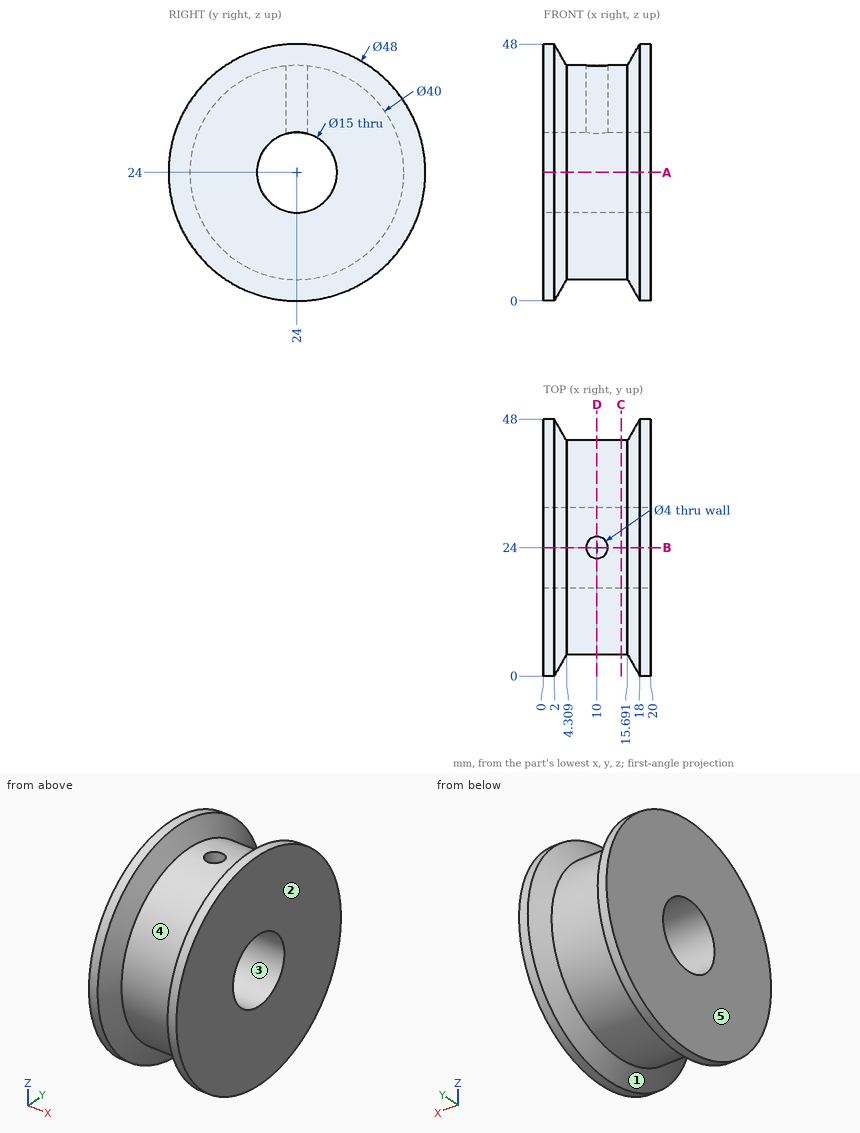
Answer from the drawing. Dimensions are ordinates in mm from the lowest x, y and z of the part. A direction names the side the tool comes from. Round coordinates to 2 decimals unless told otherwise and drop trailing zeros. Write each loop counter-clockwise with the first axis right and the second up, starting at its lowest first coordinate (ties: lowest second). Pieces come first, ordered by that corner, then holes. Notation, with made-up numbers: M 46.5,67 L 103.5,67 A5 ccw 103.5,73 Z; hole C 65.25,-8 d3. An arc over 180 degrees is marked long. Write each question's results on one line, items separated by ' | '. Start each with the question number.
Item 1: Find section C-C on x = 14.5. Write down the section's boundary in (y, z), and give its area (3 significant figures).
Item 2: Which of the six approach directions +Z, -Z, +X, -X, +Y, -Y give full straight-line access (tool end or side, diameter ignored) to the marked faces 4 and 5?
Item 3: The mould has two halves that part along Y. Classify the marked faces 1, 2 and 3: +Y half, -Y half, draft (parallel to the pull), parting line (faces both ways), or undercut.
Item 4: Given pin 1 Ø8 at (x, z) = (9, 33) entering from +Y (1 decimal); pin 2 Ø10 at (x, z) = (11, 10) entering from +Y; pin 3 Ø6.5 at (x, y) = (10, 24) entering from +Z, each flat-ended and moving along its own axis, determine where each tip first touches the part or whether it passes through.
Item 5: Find section D-D on x = 10. Write down the section's boundary in (y, z).
Item 6: Find section B-B on y = 24. Write down the section's boundary in (x, z).
Item 7: Straight lines are drawn through the part: probe 1 along X at (y, z) = (24, 34); probe 2 along Z at (x, y) = (6.25, 24); probe 3 along Z at (x, y) = (16, 26.5) (1 decimal). For each, find the intervals that lie inside material, in ascending order.
Item 8: Find section A-A on z = 24. Write down the section's boundary in (x, y).
Answer block:
1) outline: C 24,24 d40; hole C 24,24 d15 | area: 1,080 mm²
2) face 4: none | face 5: +Z, -Z, -X, +Y, -Y
3) face 1: parting line | face 2: draft | face 3: undercut
4) pin 1: stops at y = 43.4 | pin 2: stops at y = 41.86 | pin 3: stops at z = 44
5) outline: M 22,31.23 L 22,43.9 A20 ccw long 26,43.9 L 26,31.23 A7.5 cw long Z
6) outline: M 0,0 L 2,0 L 4.31,4 L 15.69,4 L 18,0 L 20,0 L 20,16.5 L 0,16.5 Z; M 0,31.5 L 8,31.5 L 8,44 L 4.31,44 L 2,48 L 0,48 Z; M 12,31.5 L 20,31.5 L 20,48 L 18,48 L 15.69,44 L 12,44 Z
7) probe 1: x = 0 to 8, 12 to 20 | probe 2: z = 4 to 16.5, 31.5 to 44 | probe 3: z = 3.6 to 16.9, 31.1 to 44.4
8) outline: M 0,0 L 2,0 L 4.31,4 L 15.69,4 L 18,0 L 20,0 L 20,16.5 L 0,16.5 Z; M 0,31.5 L 20,31.5 L 20,48 L 18,48 L 15.69,44 L 4.31,44 L 2,48 L 0,48 Z
